Geometry check sheet. Reference: the model listing, model coordinates, mm. A direction names the side the tool comes from. Coordinates: 2 decimals unless noted, no trailing zeros. Order: outer loops, then holes, each group sorted by start corner. A loop starts at its lowest first (then second) coordinate and runs counter-clockwise, first axis right, second up. Notation, with made-up numbers: (1.25, -8.75) - (17.25, -8.75) arc R19 cw to (17.25, 16.25) - close; hole circle Ø7 at (32, 39.5). An arc over 180 degrees is marked (long way). Return JSON: item names as keys, results as strings. Group by question number.
Item 1: Scan lines: probe 1 along Y at (x, z) = (0, 17.6); probe 2 along Y at (x, z) = (0, 31.25); probe 3 along Y at (x, z) = (-6.25, 17). Record each from-to range of solid material in increasing order.
Item 2: Section check C-C on z = 12. Enter the section's corners in (x, y), then the cut area to 3 significant figures.
Item 3: Tool access check on faces 4 (the cylindrical face through (-6, 0, 27)), 5 (the cylindrical face through (-6, 0, 8)), 6 (the flat face through (4, -6, 35)). Record the directions out of +Z, -Z, +X, -X, +Y, -Y that give a thin tool (end or side, any length) a straight path to the whole face; none if there is none.
Item 4: Draft check along X on faces 1 (the cylindrical face through (-1.08, -4.88, 17.52)), 2 (the cylindrical face through (-1.73, -7.81, 17.26)), 3 (the flat face through (4, -6, 0)). Enter one of: pulls with the +X half, pulls with the -X half, needs draft (parallel to the pull), parting line crosses it, or undercut.
Item 5: Section check A-A on x = 0. Enter the section's corners in (y, z), then the cut area to 3 significant figures.
Item 6: Gauge pin test, flat ends, axial feed: pin 1 (5 mm diameter, centred on x = -4, z = 4, fed in from -Y); pin 2 (6 mm diameter, centred on x = 2.5, y = 3, fed in from -Z); pin 3 (1 mm diameter, centred on y = -5, z = 24, fed in from +X). Record the tip position at first contact, or that the pin passes through.
from build123d import *

# Parameters (mm, degrees)
SKETCH_R        = 8
PAD_DEPTH       = 35
SKETCH001_R     = 5
POCKET_DEPTH    = 35.001
SKETCH002_R     = 6
POCKET001_DEPTH = 15
SKETCH003_R     = 6
POCKET002_DEPTH = 15
CHAMFER_SIZE    = 0.9
CHAMFER001_SIZE = 1


with BuildPart() as part:
    # Sketch → Pad (new body)
    with BuildSketch(Plane.XY):
        Circle(SKETCH_R)
    extrude(amount=PAD_DEPTH)

    # Sketch001 (on Face3 of Pad) → Pocket (cut, through all)
    with BuildSketch(Plane.XY.offset(35)):
        Circle(SKETCH001_R)
    extrude(amount=-POCKET_DEPTH, mode=Mode.SUBTRACT)

    # Sketch002 (on Face3 of Pocket) → Pocket001 (cut)
    with BuildSketch(Plane.XY.offset(35)):
        Circle(SKETCH002_R)
    extrude(amount=-POCKET001_DEPTH, mode=Mode.SUBTRACT)

    # Sketch003 (on Face2 of Pocket001) → Pocket002 (cut)
    with BuildSketch(Plane(origin=(0, 0, 0), x_dir=(1, 0, 0), z_dir=(0, 0, -1))):
        Circle(SKETCH003_R)
    extrude(amount=-POCKET002_DEPTH, mode=Mode.SUBTRACT)

    # Chamfer
    chamfer_edges = [part.edges().sort_by_distance(p)[0] for p in [
        (-5, 0, 15),
        (-5, 0, 20),
    ]]
    chamfer(chamfer_edges, length=CHAMFER_SIZE)

    # Chamfer001
    chamfer001_edges = [part.edges().sort_by_distance(p)[0] for p in [
        (-6, 0, 0),
        (-6, 0, 35),
    ]]
    chamfer(chamfer001_edges, length=CHAMFER001_SIZE)


solid = part.part
Computed:
{
 "1": {"probe 1": "y = -8 to -5, 5 to 8", "probe 2": "y = -8 to -6, 6 to 8", "probe 3": "y = -4.99 to 4.99"},
 "2": {"outline": "circle Ø16 at (0, 0); hole circle Ø12 at (0, 0)", "area": "88.0 mm²"},
 "3": {"face 4": "+Z", "face 5": "-Z", "face 6": "+Z, +X, -X, +Y, -Y"},
 "4": {"face 1": "undercut", "face 2": "parting line crosses it", "face 3": "needs draft"},
 "5": {"outline": "(-8, 0) - (-7, 0) - (-6, 1) - (-6, 15) - (-5.9, 15) - (-5, 15.9) - (-5, 19.1) - (-5.9, 20) - (-6, 20) - (-6, 34) - (-7, 35) - (-8, 35) - close; (5, 15.9) - (5.9, 15) - (6, 15) - (6, 1) - (7, 0) - (8, 0) - (8, 35) - (7, 35) - (6, 34) - (6, 20) - (5.9, 20) - (5, 19.1) - close", "area": "146 mm²"},
 "6": {"pin 1": "stops at y = -7.86", "pin 2": "stops at z = 0.09", "pin 3": "stops at x = 6.61"}
}
